```python
from build123d import *

# Parameters (mm, degrees)
SKETCH1_W           = 58
SKETCH1_H           = 38
SKETCH1_R           = 7
SKETCH1_R_2         = 1.65
BOSS_EXTRUDE1_DEPTH = 6.35
FILLET1_R           = 4
CUT_EXTRUDE1_DEPTH  = 65.127392743
SKETCH3_R           = 1.35
CUT_EXTRUDE2_DEPTH  = 65.127392743


with BuildPart() as part:
    # Sketch1 → Boss-Extrude1 (new body)
    with BuildSketch(Plane(origin=(0, 0, 0), x_dir=(1, 0, 0), z_dir=(0, 1, 0))):
        with Locations((25, 15)):
            Rectangle(SKETCH1_W, SKETCH1_H)
        with Locations(Location((25, 15, 0), (0, 0, 270))):
            Circle(SKETCH1_R, mode=Mode.SUBTRACT)
        with Locations(Location((0, 30, 0), (0, 0, 270))):
            Circle(SKETCH1_R_2, mode=Mode.SUBTRACT)
        with Locations(Location((50, 30, 0), (0, 0, 270))):
            Circle(SKETCH1_R_2, mode=Mode.SUBTRACT)
        with Locations(Location((50, 0, 0), (0, 0, 270))):
            Circle(SKETCH1_R_2, mode=Mode.SUBTRACT)
        with Locations(Location((0, 0, 0), (0, 0, 270))):
            Circle(SKETCH1_R_2, mode=Mode.SUBTRACT)
    extrude(amount=BOSS_EXTRUDE1_DEPTH)

    # Fillet1
    fillet1_edges = [part.edges().sort_by_distance(p)[0] for p in [
        (-4, 3.175, -34),
        (54, 3.175, -34),
        (54, 3.175, 4),
        (-4, 3.175, 4),
    ]]
    fillet(fillet1_edges, radius=FILLET1_R)

    # Sketch2 → Cut-Extrude1 (cut, through all)
    with BuildSketch(Plane(origin=(0, 6.35, 0), x_dir=(1, 0, 0), z_dir=(0, 1, 0))):
        with BuildLine():
            Line((24, 24.250000018), (26, 24.250000018))
            ThreePointArc((26, 24.250000018), (26.75, 23.500000018), (26, 22.750000018))
            Line((26, 22.750000018), (24, 22.750000018))
            ThreePointArc((24, 22.750000018), (23.25, 23.500000018), (24, 24.250000018))
        make_face()
        with BuildLine():
            Line((24, 5.749999982), (26, 5.749999982))
            ThreePointArc((26, 5.749999982), (26.75, 6.499999982), (26, 7.249999982))
            Line((26, 7.249999982), (24, 7.249999982))
            ThreePointArc((24, 7.249999982), (23.25, 6.499999982), (24, 5.749999982))
        make_face()
    extrude(amount=-CUT_EXTRUDE1_DEPTH, mode=Mode.SUBTRACT)

    # Sketch3 → Cut-Extrude2 (cut, through all)
    with BuildSketch(Plane(origin=(0, 6.35, 0), x_dir=(1, 0, 0), z_dir=(0, 1, 0))):
        with Locations(Location((35.606601718, 25.606601718, 0), (0, 0, 270))):
            Circle(SKETCH3_R)
        with Locations(Location((35.606601718, 4.393398282, 0), (0, 0, 270))):
            Circle(SKETCH3_R)
        with Locations(Location((14.393398282, 25.606601718, 0), (0, 0, 270))):
            Circle(SKETCH3_R)
        with Locations(Location((14.393398282, 4.393398282, 0), (0, 0, 270))):
            Circle(SKETCH3_R)
    extrude(amount=-CUT_EXTRUDE2_DEPTH, mode=Mode.SUBTRACT)


solid = part.part
```
Input: part model. Units: mm. Frame: model coordinates. A direction names the side the tool comes from. Round coordinates to 2 decimals unless told otherwise and drop trailing zeros. Order: outer loops, then holes, each group sorted by start corner. A loop starts at its lowest first (then second) coordinate and runs counter-clockwise, first axis right, second up. Notation, with made-up numbers: (10, -3.5) - (66, -3.5) arc R3 cw to (66, 0.5) - close; hole circle Ø6 at (39, -7). An arc over 180 degrees is marked (long way). Answer in a Markdown table with one row per item.
Item 1: Line query: line 1 (X direction, y = 5, z = -30); line 2 (X direction, y = 6.25, z = -6.5); line 3 (X direction, y = 5.75, z = -15). Output: solid intervals per line, ascending.
Model answer:
| item | result |
|---|---|
| line 1 | x = -4 to -1.65, 1.65 to 48.35, 51.65 to 54 |
| line 2 | x = -4 to 23.25, 26.75 to 54 |
| line 3 | x = -4 to 18, 32 to 54 |
Item 2: Section query D-D (y = 3.25). Give the number of separate pieces and of enclosed holes in the cut face, then the cut area to 3 significant figures.
Model answer:
| item | result |
|---|---|
| separate pieces | 1 |
| enclosed holes | 11 |
| area | 1,970 mm² |
Item 3: Section query A-A (x = 25). Return the cut outline in (y, z).
Model answer:
| item | result |
|---|---|
| outline | (0, -34) - (6.35, -34) - (6.35, -24.25) - (0, -24.25) - close; (0, -22.75) - (6.35, -22.75) - (6.35, -22) - (0, -22) - close; (0, -8) - (6.35, -8) - (6.35, -7.25) - (0, -7.25) - close; (0, -5.75) - (6.35, -5.75) - (6.35, 4) - (0, 4) - close |
Item 4: Pin query (flat end, axial travel): pin 1 (1.6 mm diameter, centred on x = 35.61, z = -25.61, fed in from +Y). Return the tip coordinate at first contact, or that it passes through.
Model answer:
| item | result |
|---|---|
| pin 1 | passes through |
Item 5: Section query B-B (z = -15). Return the cut outline in (x, y).
Model answer:
| item | result |
|---|---|
| outline | (-4, 0) - (18, 0) - (18, 6.35) - (-4, 6.35) - close; (32, 0) - (54, 0) - (54, 6.35) - (32, 6.35) - close |
Item 6: Section query C-C (z = -4). Return the cut outline in (x, y), then the cut area to 3 significant figures.
Model answer:
| item | result |
|---|---|
| outline | (-4, 0) - (13.1, 0) - (13.1, 6.35) - (-4, 6.35) - close; (15.68, 0) - (34.32, 0) - (34.32, 6.35) - (15.68, 6.35) - close; (36.9, 0) - (54, 0) - (54, 6.35) - (36.9, 6.35) - close |
| area | 335 mm² |
Item 7: Mould query, pull axis X, two halves, no side actions, for faces 1 (the flat face through (54, 3, -15)), 2 (the flat face through (25, 3, -34)), 3 (the cylindrical face through (23.25, 3.22, -6.52)), 4 (the cylindrical face through (-2.859, 3.219, -32.797)). Classes: released by +X, released by -X, zero draft, split by the parting line, or undercut.
Model answer:
| item | result |
|---|---|
| face 1 | released by +X |
| face 2 | zero draft |
| face 3 | undercut |
| face 4 | released by -X |
Item 8: Reachability of faces 5 (the cylindrical face through (-2.859, 3.219, 2.797)), 6 (the flat face through (25, 3, -22.75)) from +Z, -Z, +X, -X, +Y, -Y: full face, straight path, thin tool, end or side. Return the list, or none.
Model answer:
| item | result |
|---|---|
| face 5 | +Z, -X, +Y, -Y |
| face 6 | +Y, -Y |
